Geometry check sheet. Reference: the model listing, model coordinates, mm. Face numbers are marked on the shaded views. Coordinates: 2 decimals unless noted, no trailing zeros. Order: outer loops, then holes, each group sorted by start corner. A loop starts at its lowest first (then second) coordinate and runs counter-clockwise, first axis right, second up. Notation, with made-up numbers: M -38,24 L -17,24 A12 cw -17,43 Z; hole C 55.5,-16.75 d2. An arc over 180 degrees is marked long. One line per item, written item: value. Start each with the question number.
1) Sectioned sample at B-B, the plane y = -51. Enter the section's corners in (x, z).
2) Draft check along Y on the marked faces 1 and 2. Enter one of: pulls with the +Y half, pulls with the -Y half, needs draft (parallel to the pull), parting line crosses it, or undercut.
3) Go/stop test with flat-tipped pins: P1, Ø5, axis at x = 28, y = -1, coming from the -Z side; P2, Ø1.8, axis at x = -81.5, y = 59, coming from the +Z side. Record where each tip stops, or that it passes through.
4) Thickness scan on L1, parallel to Y at x = 81.5, z = 33.25; L2, parallel to X at y = 59, z = 36.5; L3, parallel to X at y = -25.5, z = 35.5. Record the ranges inside material, lowest first. Write a range as from..to.
5) Sectioned sample at A-A, the plane z = 33. Enter the section's corners in (x, y).
6) Sectioned sample at C-C, the plane x = -23.5. Enter the section's corners in (y, z).
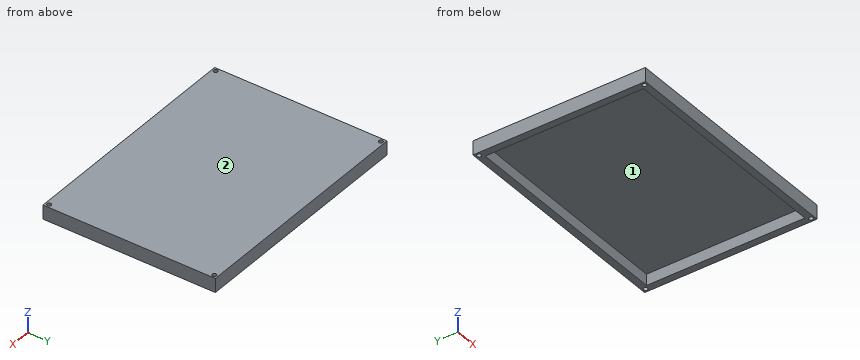
```python
from build123d import *

# Parameters (mm, degrees)
SKETCH013_W               = 160
SKETCH013_H               = 115
EXTRUDE013_DEPTH          = 2
SKETCH012_W               = 168
SKETCH012_H               = 123
SKETCH012_R               = 1.5
SKETCH012_W_2             = 158
SKETCH012_H_2             = 113
EXTRUDE012_DEPTH          = 10
FUSION003_PLACEMENT_ANGLE = 180


with BuildPart() as extrude013:
    # Sketch013 → Extrude013 (new body)
    with BuildSketch(Plane.XY):
        Rectangle(SKETCH013_W, SKETCH013_H)
    extrude(amount=EXTRUDE013_DEPTH)


with BuildPart() as fusion003:
    # Sketch012 → Extrude012 (new body)
    with BuildSketch(Plane.XY):
        Rectangle(SKETCH012_W, SKETCH012_H)
        with Locations((-81.5, 59)):
            Circle(SKETCH012_R, mode=Mode.SUBTRACT)
        with Locations((81.5, 59)):
            Circle(SKETCH012_R, mode=Mode.SUBTRACT)
        with Locations((81.5, -59)):
            Circle(SKETCH012_R, mode=Mode.SUBTRACT)
        with Locations((-81.5, -59)):
            Circle(SKETCH012_R, mode=Mode.SUBTRACT)
        Rectangle(SKETCH012_W_2, SKETCH012_H_2, mode=Mode.SUBTRACT)
    extrude(amount=EXTRUDE012_DEPTH)

    # Fusion003: union Extrude013
    add(extrude013.part)


with BuildPart() as fusion003_1:
    # Fusion003 placement: moved
    add(fusion003.part.moved(Location((0, 0, 39.5))).rotate(Axis((0, 0, 39.5), (1, 0, 0)), FUSION003_PLACEMENT_ANGLE))


solid = fusion003_1.part
```
Final values:
1. outline: M -84,29.5 L -79,29.5 L -79,37.5 L 79,37.5 L 79,29.5 L 84,29.5 L 84,39.5 L -84,39.5 Z
2. face 1: undercut
2. face 2: needs draft
3. P1: stops at z = 37.5
3. P2: passes through
4. L1: y = -61.5..-60.5, -57.5..57.5, 60.5..61.5
4. L2: x = -84..-83, -80..80, 83..84
4. L3: x = -84..-79, 79..84
5. outline: M -84,-61.5 L 84,-61.5 L 84,61.5 L -84,61.5 Z; hole C -81.5,-59 d3; hole C -81.5,59 d3; hole M -79,-56.5 L 79,-56.5 L 79,56.5 L -79,56.5 Z; hole C 81.5,-59 d3; hole C 81.5,59 d3
6. outline: M -61.5,29.5 L -56.5,29.5 L -56.5,37.5 L 56.5,37.5 L 56.5,29.5 L 61.5,29.5 L 61.5,39.5 L -61.5,39.5 Z
